For this review, take the finished solid that the model builds, in its own axes (mm). Round coordinates to 2 decimals unless told otherwise and drop trailing zeros. Order: outer loops, then holes, each group sorted by start corner. A loop starts at its lowest first (then second) coordinate and runs counter-clockwise, first axis right, second up. Notation, with made-up numbers: M 85,56 L 93,56 A14 ccw 93,63 Z; hole C -23.5,12 d8. An arc over 180 degrees is marked long. Answer as a JSON object with one key per item and string values.
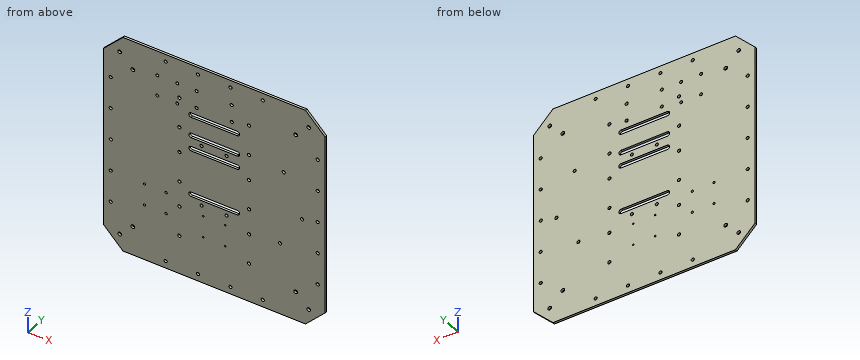
from build123d import *

# Parameters (mm, degrees)
BOSS_EXTRUDE1_DEPTH = 3.175
SKETCH2_R           = 2.159
CUT_EXTRUDE1_DEPTH  = 297.247830215
CUT_EXTRUDE2_DEPTH  = 297.247830215
SKETCH7_R           = 1.524
CUT_EXTRUDE3_DEPTH  = 297.247830215
SKETCH10_R          = 2.159
CUT_EXTRUDE6_DEPTH  = 297.247830215
SKETCH9_R           = 2.032
CUT_EXTRUDE5_DEPTH  = 297.247830215
SKETCH13_R          = 1.1
CUT_EXTRUDE8_DEPTH  = 297.247830215
SKETCH14_R          = 2.54
CUT_EXTRUDE9_DEPTH  = 297.247830215
SKETCH15_R          = 2.159
CUT_EXTRUDE10_DEPTH = 297.247830215
SKETCH16_R          = 2.159
CUT_EXTRUDE11_DEPTH = 297.247830215
SKETCH17_R          = 2.2225
CUT_EXTRUDE13_DEPTH = 297.247830215


with BuildPart() as part:
    # Sketch1 → Boss-Extrude1 (new body)
    with BuildSketch(Plane(origin=(0, 0, 0), x_dir=(1, 0, 0), z_dir=(0, 1, 0))):
        Polygon((-94.345284264, 72.258976948), (-121.286052627, 45.318208585), (-121.286052627, -205.600254688), (-94.345284264, -232.541023052), (156.573179009, -232.541023052), (183.513947373, -205.600254688), (183.513947373, 45.318208585), (156.573179009, 72.258976948), align=None)
    extrude(amount=BOSS_EXTRUDE1_DEPTH)

    # Sketch2 → Cut-Extrude1 (cut, through all)
    with BuildSketch(Plane(origin=(0, 3.175, 0), x_dir=(1, 0, 0), z_dir=(0, 1, 0))):
        with Locations(Location((13.841947373, -37.469023052, 0), (0, 0, 270))):
            Circle(SKETCH2_R)
        with Locations(Location((48.131947373, -37.469023052, 0), (0, 0, 270))):
            Circle(SKETCH2_R)
        with Locations(Location((13.841947373, -122.559023052, 0), (0, 0, 270))):
            Circle(SKETCH2_R)
        with Locations(Location((48.131947373, -122.559023052, 0), (0, 0, 270))):
            Circle(SKETCH2_R)
    extrude(amount=-CUT_EXTRUDE1_DEPTH, mode=Mode.SUBTRACT)

    # Sketch4 → Cut-Extrude2 (cut, through all)
    with BuildSketch(Plane(origin=(0, 3.175, 0), x_dir=(1, 0, 0), z_dir=(0, 1, 0))):
        with BuildLine():
            Line((-0.636052627, -44.466023052), (62.863947373, -44.466023052))
            ThreePointArc((62.863947373, -44.466023052), (66.038947373, -47.641023052), (62.863947373, -50.816023052))
            Line((62.863947373, -50.816023052), (-0.636052627, -50.816023052))
            ThreePointArc((-0.636052627, -50.816023052), (-3.811052627, -47.641023052), (-0.636052627, -44.466023052))
        make_face()
        with BuildLine():
            Line((-0.636052627, -109.466023052), (62.863947373, -109.466023052))
            ThreePointArc((62.863947373, -109.466023052), (66.038947373, -112.641023052), (62.863947373, -115.816023052))
            Line((62.863947373, -115.816023052), (-0.636052627, -115.816023052))
            ThreePointArc((-0.636052627, -115.816023052), (-3.811052627, -112.641023052), (-0.636052627, -109.466023052))
        make_face()
        with BuildLine():
            Line((-0.636052627, -128.401023052), (62.863947373, -128.401023052))
            ThreePointArc((62.863947373, -128.401023052), (66.038947373, -131.576023052), (62.863947373, -134.751023052))
            Line((62.863947373, -134.751023052), (-0.636052627, -134.751023052))
            ThreePointArc((-0.636052627, -134.751023052), (-3.811052627, -131.576023052), (-0.636052627, -128.401023052))
        make_face()
        with BuildLine():
            Line((-0.636052627, -157.401023052), (62.863947373, -157.401023052))
            ThreePointArc((62.863947373, -157.401023052), (66.038947373, -160.576023052), (62.863947373, -163.751023052))
            Line((62.863947373, -163.751023052), (-0.636052627, -163.751023052))
            ThreePointArc((-0.636052627, -163.751023052), (-3.811052627, -160.576023052), (-0.636052627, -157.401023052))
        make_face()
    extrude(amount=-CUT_EXTRUDE2_DEPTH, mode=Mode.SUBTRACT)

    # Sketch7 → Cut-Extrude3 (cut, through all)
    with BuildSketch(Plane(origin=(0, 3.175, 0), x_dir=(1, 0, 0), z_dir=(0, 1, 0))):
        with Locations(Location((-34.926052627, -5.719023052, 0), (0, 0, 270))):
            Circle(SKETCH7_R)
        with Locations(Location((-34.926052627, -35.691023052, 0), (0, 0, 270))):
            Circle(SKETCH7_R)
        with Locations(Location((-64.898052627, -35.691023052, 0), (0, 0, 90))):
            Circle(SKETCH7_R)
        with Locations(Location((-64.898052627, -5.719023052, 0), (0, 0, 90))):
            Circle(SKETCH7_R)
    extrude(amount=-CUT_EXTRUDE3_DEPTH, mode=Mode.SUBTRACT)

    # Sketch10 → Cut-Extrude6 (cut, through all)
    with BuildSketch(Plane.XZ):
        with Locations(Location((6.983947373, 198.041023052, 0), (0, 0, 270))):
            Circle(SKETCH10_R)
        with Locations(Location((55.243947373, 198.041023052, 0), (0, 0, 270))):
            Circle(SKETCH10_R)
        with Locations(Location((6.983947373, 173.911023052, 0), (0, 0, 270))):
            Circle(SKETCH10_R)
        with Locations(Location((55.243947373, 173.911023052, 0), (0, 0, 270))):
            Circle(SKETCH10_R)
    extrude(amount=-CUT_EXTRUDE6_DEPTH, mode=Mode.SUBTRACT)

    # Sketch9 → Cut-Extrude5 (cut, through all)
    with BuildSketch(Plane(origin=(0, 0, 0), x_dir=(-1, 0, 0), z_dir=(0, -1, 0))):
        with Locations(Location((47.118052627, -197.997023052, 0), (0, 0, 90))):
            Circle(SKETCH9_R)
        with Locations(Location((19.686052627, -197.997023052, 0), (0, 0, 270))):
            Circle(SKETCH9_R)
        with Locations(Location((47.118052627, -169.041023052, 0), (0, 0, 90))):
            Circle(SKETCH9_R)
        with Locations(Location((19.686052627, -169.041023052, 0), (0, 0, 270))):
            Circle(SKETCH9_R)
    extrude(amount=-CUT_EXTRUDE5_DEPTH, mode=Mode.SUBTRACT)

    # Sketch13 → Cut-Extrude8 (cut, through all)
    with BuildSketch(Plane.XZ):
        with Locations(Location((16.113947373, 22.991023052, 0), (0, 0, 270))):
            Circle(SKETCH13_R)
        with Locations(Location((16.113947373, -7.008976948, 0), (0, 0, 270))):
            Circle(SKETCH13_R)
        with Locations(Location((46.113947373, -7.008976948, 0), (0, 0, 90))):
            Circle(SKETCH13_R)
        with Locations(Location((46.113947373, 22.991023052, 0), (0, 0, 90))):
            Circle(SKETCH13_R)
    extrude(amount=-CUT_EXTRUDE8_DEPTH, mode=Mode.SUBTRACT)

    # Sketch14 → Cut-Extrude9 (cut, through all)
    with BuildSketch(Plane.XZ):
        with Locations(Location((-98.835412325, 210.090382749, 0), (0, 0, 270))):
            Circle(SKETCH14_R)
        with Locations(Location((-80.874900083, 192.129870507, 0), (0, 0, 270))):
            Circle(SKETCH14_R)
        with Locations(Location((143.102794828, 192.129870507, 0), (0, 0, 90))):
            Circle(SKETCH14_R)
        with Locations(Location((161.06330707, 210.090382749, 0), (0, 0, 90))):
            Circle(SKETCH14_R)
        with Locations(Location((-98.835412325, -49.808336646, 0), (0, 0, 90))):
            Circle(SKETCH14_R)
        with Locations(Location((-80.874900083, -31.847824404, 0), (0, 0, 90))):
            Circle(SKETCH14_R)
        with Locations(Location((161.06330707, -49.808336646, 0), (0, 0, 270))):
            Circle(SKETCH14_R)
        with Locations(Location((143.102794828, -31.847824404, 0), (0, 0, 270))):
            Circle(SKETCH14_R)
    extrude(amount=-CUT_EXTRUDE9_DEPTH, mode=Mode.SUBTRACT)

    # Sketch15 → Cut-Extrude10 (cut, through all)
    with BuildSketch(Plane.XZ):
        with Locations(Location((8.888947373, 222.381023052, 0), (0, 0, 270))):
            Circle(SKETCH15_R)
        with Locations(Location((-35.561052627, 222.381023052, 0), (0, 0, 270))):
            Circle(SKETCH15_R)
        with Locations(Location((-111.126052627, 80.141023052, 0), (0, 0, 270))):
            Circle(SKETCH15_R)
        with Locations(Location((-111.126052627, 124.591023052, 0), (0, 0, 270))):
            Circle(SKETCH15_R)
        with Locations(Location((-111.126052627, 169.041023052, 0), (0, 0, 270))):
            Circle(SKETCH15_R)
        with Locations(Location((173.353947373, 169.041023052, 0), (0, 0, 90))):
            Circle(SKETCH15_R)
        with Locations(Location((173.353947373, 124.591023052, 0), (0, 0, 90))):
            Circle(SKETCH15_R)
        with Locations(Location((173.353947373, 80.141023052, 0), (0, 0, 90))):
            Circle(SKETCH15_R)
        with Locations(Location((97.788947373, 222.381023052, 0), (0, 0, 90))):
            Circle(SKETCH15_R)
        with Locations(Location((53.338947373, 222.381023052, 0), (0, 0, 90))):
            Circle(SKETCH15_R)
        with Locations(Location((53.338947373, -62.098976948, 0), (0, 0, 270))):
            Circle(SKETCH15_R)
        with Locations(Location((97.788947373, -62.098976948, 0), (0, 0, 270))):
            Circle(SKETCH15_R)
        with Locations(Location((173.353947373, 35.691023052, 0), (0, 0, 270))):
            Circle(SKETCH15_R)
        with Locations(Location((173.353947373, -8.758976948, 0), (0, 0, 270))):
            Circle(SKETCH15_R)
        with Locations(Location((-111.126052627, -8.758976948, 0), (0, 0, 90))):
            Circle(SKETCH15_R)
        with Locations(Location((-111.126052627, 35.691023052, 0), (0, 0, 90))):
            Circle(SKETCH15_R)
        with Locations(Location((-35.561052627, -62.098976948, 0), (0, 0, 90))):
            Circle(SKETCH15_R)
        with Locations(Location((8.888947373, -62.098976948, 0), (0, 0, 90))):
            Circle(SKETCH15_R)
    extrude(amount=-CUT_EXTRUDE10_DEPTH, mode=Mode.SUBTRACT)

    # Sketch16 → Cut-Extrude11 (cut, through all)
    with BuildSketch(Plane(origin=(0, 0, 0), x_dir=(-1, 0, 0), z_dir=(0, -1, 0))):
        with Locations(Location((-126.617947373, -131.830023052, 0), (0, 0, 90))):
            Circle(SKETCH16_R)
        with Locations(Location((-121.537947373, -28.452023052, 0), (0, 0, 90))):
            Circle(SKETCH16_R)
        with Locations(Location((-151.763947373, -75.274023052, 0), (0, 0, 90))):
            Circle(SKETCH16_R)
    extrude(amount=-CUT_EXTRUDE11_DEPTH, mode=Mode.SUBTRACT)

    # Sketch17 → Cut-Extrude13 (cut, through all)
    with BuildSketch(Plane(origin=(0, 3.175, 0), x_dir=(1, 0, 0), z_dir=(0, 1, 0))):
        with Locations(Location((78.992947373, -178.566023052, 0), (0, 0, 270))):
            Circle(SKETCH17_R)
        with Locations(Location((-16.765052627, -178.566023052, 0), (0, 0, 270))):
            Circle(SKETCH17_R)
        with Locations(Location((78.992947373, -136.656023052, 0), (0, 0, 270))):
            Circle(SKETCH17_R)
        with Locations(Location((-16.765052627, -136.656023052, 0), (0, 0, 270))):
            Circle(SKETCH17_R)
        with Locations(Location((78.992947373, -101.096023052, 0), (0, 0, 270))):
            Circle(SKETCH17_R)
        with Locations(Location((-16.765052627, -101.096023052, 0), (0, 0, 270))):
            Circle(SKETCH17_R)
        with Locations(Location((78.992947373, -59.186023052, 0), (0, 0, 270))):
            Circle(SKETCH17_R)
        with Locations(Location((-16.765052627, -59.186023052, 0), (0, 0, 270))):
            Circle(SKETCH17_R)
        with Locations(Location((78.992947373, -23.626023052, 0), (0, 0, 270))):
            Circle(SKETCH17_R)
        with Locations(Location((-16.765052627, -23.626023052, 0), (0, 0, 270))):
            Circle(SKETCH17_R)
        with Locations(Location((78.992947373, 18.283976948, 0), (0, 0, 270))):
            Circle(SKETCH17_R)
        with Locations(Location((-16.765052627, 18.283976948, 0), (0, 0, 270))):
            Circle(SKETCH17_R)
    extrude(amount=-CUT_EXTRUDE13_DEPTH, mode=Mode.SUBTRACT)


solid = part.part
1) Insertion check: P1, Ø2.5, axis at x = -111.13, z = 169.04, coming from the -Y side. The pin has a flat end and moves straight along its axis. Give the tip position at first contact, or say it passes through.
Geometry check:
{"P1": "passes through"}
2) Add section B-B on y = 2.3. State how many separate pieces and enclosed holes the cut face has, and give its area (3 significant figures).
Geometry check:
{"separate pieces": "1", "enclosed holes": "65", "area": "88,800 mm²"}
3) For L1, parallel to X at y = 0.35, z = 178; L2, parallel to Z at x = 22.5, y = 0.3; L3, parallel to X at y = 0.35, z = 79.5, list the stretches that pass through material, from the lowest coordinate up.
Geometry check:
{"L1": "x = -121.29 to -18.91, -14.62 to 76.84, 81.14 to 183.51", "L2": "z = -72.26 to 44.47, 50.82 to 109.47, 115.82 to 128.4, 134.75 to 157.4, 163.75 to 232.54", "L3": "x = -121.29 to -113.19, -109.06 to 171.29, 175.42 to 183.51"}
4) Add section A-A on x = 35. State the section outline as (y, z) points (3 decimals).
Geometry check:
{"outline": "M 0,-72.259 L 3.175,-72.259 L 3.175,44.466 L 0,44.466 Z; M 0,50.816 L 3.175,50.816 L 3.175,109.466 L 0,109.466 Z; M 0,115.816 L 3.175,115.816 L 3.175,128.401 L 0,128.401 Z; M 0,134.751 L 3.175,134.751 L 3.175,157.401 L 0,157.401 Z; M 0,163.751 L 3.175,163.751 L 3.175,232.541 L 0,232.541 Z"}
